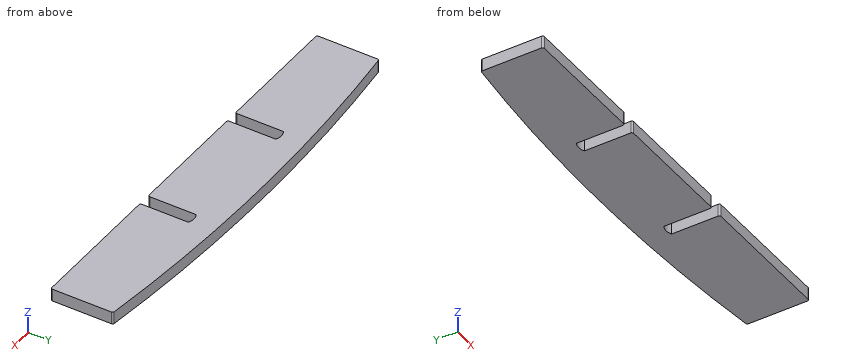
from build123d import *

# Parameters (mm, degrees)
RESSALTO_EXTRUS_O1_DEPTH = 2


with BuildPart() as part:
    # Esboço1 → Ressalto-extrusão1 (new body)
    with BuildSketch(Plane.XY):
        with BuildLine():
            Line((-9.717847221, -7.732050808), (9.717847221, -7.732050808))
            ThreePointArc((9.717847221, -7.732050808), (9.917359364, -7.649410172), (10, -7.449898029))
            Line((10, -7.449898029), (10, 0))
            ThreePointArc((10, 0), (11, 0.267949192), (12, 0))
            Line((12, 0), (12, -7.449898029))
            ThreePointArc((12, -7.449898029), (12.082640636, -7.649410172), (12.282152779, -7.732050808))
            Line((12.282152779, -7.732050808), (34.217847221, -7.732050808))
            ThreePointArc((34.217847221, -7.732050808), (34.417359364, -7.649410172), (34.5, -7.449898029))
            Line((34.5, -7.449898029), (34.5, 2.017476071))
            ThreePointArc((34.5, 2.017476071), (34.428811399, 2.204837503), (34.251168098, 2.297654424))
            ThreePointArc((34.251168098, 2.297654424), (1, 4.267949192), (-32.251168098, 2.297654424))
            ThreePointArc((-32.251168098, 2.297654424), (-32.428811399, 2.204837503), (-32.5, 2.017476071))
            Line((-32.5, 2.017476071), (-32.5, -7.449898029))
            ThreePointArc((-32.5, -7.449898029), (-32.417359364, -7.649410172), (-32.217847221, -7.732050808))
            Line((-32.217847221, -7.732050808), (-12.282152779, -7.732050808))
            ThreePointArc((-12.282152779, -7.732050808), (-12.082640636, -7.649410172), (-12, -7.449898029))
            Line((-12, -7.449898029), (-12, 0))
            ThreePointArc((-12, 0), (-11, 0.267949192), (-10, 0))
            Line((-10, 0), (-10, -7.449898029))
            ThreePointArc((-10, -7.449898029), (-9.917359364, -7.649410172), (-9.717847221, -7.732050808))
        make_face()
    extrude(amount=RESSALTO_EXTRUS_O1_DEPTH)


solid = part.part
Can you work these out from the model? Positions are in its coordinate system, mm. Give positions to 0.01 mm unless a question says otherwise; leave off trailing zeros. Loops run counter-clockwise (first coordinate to the right, second up) from the corner with the lowest first, then second, coordinate; pieces in that order, holes last. Notation, with made-up numbers: (2, 81.25) - (41, 81.25) arc R24 ccw to (41, 107.25) - close; hole circle Ø7 at (37.5, -30.5). An arc over 180 degrees is marked (long way). Return JSON: item names as keys, results as strings.
1. I want a section at C-C on x = 25.5. Please give me the cut outline in (y, z), and give its area (3 significant figures).
Output values:
{"outline": "(-7.73, 0) - (3.2, 0) - (3.2, 2) - (-7.73, 2) - close", "area": "21.9 mm²"}
2. If I drill on line 1 (X direction, y = -5.5, z = 1.3); line 2 (Y direction, x = 2.5, z = 1.7); line 3 (Y direction, x = 18, z = 1.7), over which ranges is the centre line in solid material (lowest first)?
Output values:
{"line 1": "x = -32.5 to -12, -10 to 10, 12 to 34.5", "line 2": "y = -7.73 to 4.26", "line 3": "y = -7.73 to 3.75"}
3. I want a section at D-D on x = -19.5. Please give me the cut outline in (y, z).
Output values:
{"outline": "(-7.73, 0) - (3.52, 0) - (3.52, 2) - (-7.73, 2) - close"}
4. I want a section at A-A on y = -4.5. Please give me the cut outline in (x, z).
Output values:
{"outline": "(-32.5, 0) - (-12, 0) - (-12, 2) - (-32.5, 2) - close; (-10, 0) - (10, 0) - (10, 2) - (-10, 2) - close; (12, 0) - (34.5, 0) - (34.5, 2) - (12, 2) - close"}
